Design review of the part built by this model. Coordinates are the model's own, in mm. Face numbers are marked on the shaded views. A direction names the side the tool comes from. Give positions to 0.01 mm unless a question says otherwise; leave off trailing zeros. Write each loop counter-clockwise with the first axis right and the second up, starting at its lowest first coordinate (ties: lowest second). Pieces come first, ordered by that corner, then holes. Notation, with made-up numbers: M 2.5,54 L 14.5,54 A14 ccw 14.5,63 Z; hole C 71,5.25 d3. An arc over 180 degrees is marked long. Use one line per item in the form item = value. Start each with the question number.
from build123d import *

# Parameters (mm, degrees)
SKETCH2_R           = 13.4112
BOSS_EXTRUDE1_DEPTH = 38.1
SKETCH5_W           = 26.8224
SKETCH5_H           = 184.15
BOSS_EXTRUDE2_DEPTH = 16.7386
SKETCH8_W           = 76.2
SKETCH8_H           = 38.1
BOSS_EXTRUDE3_DEPTH = 13.97
SKETCH9_W           = 1.016
SKETCH9_H           = 38.1
BOSS_EXTRUDE4_DEPTH = 38.1
SKETCH10_W          = 25.4
SKETCH10_H          = 38.1
BOSS_EXTRUDE5_DEPTH = 12.446
FILLET1_R           = 3.81


with BuildPart() as part:
    # Sketch2 → Boss-Extrude1 (new body)
    with BuildSketch(Plane.XY):
        with Locations(Location((0, 0, 0), (0, 0, 180))):
            Circle(SKETCH2_R)
    extrude(amount=BOSS_EXTRUDE1_DEPTH)

    # Sketch5 → Boss-Extrude2 (add)
    with BuildSketch(Plane.XY.offset(38.1)):
        with Locations((0, 92.075)):
            Rectangle(SKETCH5_W, SKETCH5_H)
    extrude(amount=-BOSS_EXTRUDE2_DEPTH)

    # Sketch8 → Boss-Extrude3 (add)
    with BuildSketch(Plane(origin=(0, 184.15, 0), x_dir=(1, 0, 0), z_dir=(0, 1, 0))):
        with Locations((0, -18.948214994)):
            Rectangle(SKETCH8_W, SKETCH8_H)
    extrude(amount=BOSS_EXTRUDE3_DEPTH)

    # Sketch9 → Boss-Extrude4 (add)
    with BuildSketch(Plane(origin=(0, 198.12, 0), x_dir=(1, 0, 0), z_dir=(0, 1, 0))):
        with Locations((-37.592, -18.948214994)):
            Rectangle(SKETCH9_W, SKETCH9_H)
        with Locations((37.592, -18.948214994)):
            Rectangle(SKETCH9_W, SKETCH9_H)
    extrude(amount=BOSS_EXTRUDE4_DEPTH)

    # Sketch10 → Boss-Extrude5 (add)
    with BuildSketch(Plane(origin=(0, 236.22, 0), x_dir=(1, 0, 0), z_dir=(0, 1, 0))):
        with Locations((-25.4, -18.948214994)):
            Rectangle(SKETCH10_W, SKETCH10_H)
        with Locations((25.4, -18.948214994)):
            Rectangle(SKETCH10_W, SKETCH10_H)
    extrude(amount=BOSS_EXTRUDE5_DEPTH)

    # Fillet1
    # the kernel refuses this fillet: 3.81 mm, written as the material it takes off along each edge
    with BuildSketch(Plane(origin=(15.598152153, 184.15, 38.1), x_dir=(0, 0, -1), z_dir=(-1, 0, 0))) as fillet1_piece_1:
        with BuildLine():
            CenterArc((3.81, 0.874780861), FILLET1_R, 180, 13.273598337)
            Line((0, 0.874780861), (-0.0762, 0.874780861))
            Line((-0.0762, 0.874780861), (-0.0762, 0))
            Line((-0.0762, 0), (0, -0.0762))
            ThreePointArc((0, -0.0762), (0.050892503, -0.0762), (0.027620706, -0.017495617))
            Line((0.027620706, -0.017495617), (0.101785006, 0))
        make_face()
    extrude(amount=31.196304306, mode=Mode.SUBTRACT)


solid = part.part
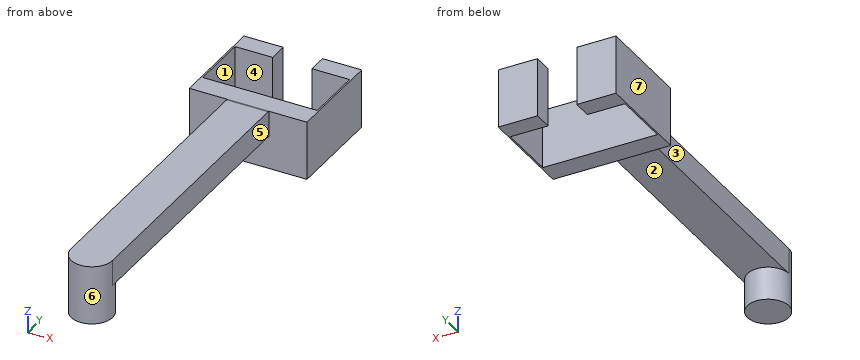
1. We need section B-B (z = 18). State the section outline as (x, y) points, and give its area (3 significant figures).
2. To check wall thickness, follow L1, parallel to Y at x = -23.5, z = 9.5; L2, parallel to X at y = 25, z = 31; L3, parallel to Y at x = 9, z = 11. State the ranges of each line that lie inside material, in increasing order.
3. For the marked faces 4, 5, 6 and 7, list the 3-axis set-ups (+Z, -Z, +X, -X, +Y, -Y) from which the entire face can be reached by the end or side of a thin tool; tool diameter is ignored.
4. We need section C-C (z = 32). State the section outline as (x, y) points.
5. We need section D-D (x = 0). State the section outline as (y, z) points.
6. We need section A-A (x = -28.5). State the section outline as (y, z) points, and give its area (3 significant figures).
7. Draft analysis for pull direction X (two halves, no side actions). For the marked faces 1, 2 and 3, state which applies: pulls with the +X half, pulls with the -X half, needs draft (parallel to the pull), parting line crosses it, or undercut.
8. Clearance check with flat-ended pins moving along their axes: pin 1 Ø6 at (y, z) = (60, 31.5) entering from +X; pin 2 Ø6 at (y, z) = (72, 24) entering from -X; pin 3 Ø12 at (x, z) = (31, 23.5) entering from -Y. State where each tip first meets the part, or that it passes through.
Answer block:
q1.outline = M -38.1,184.15 L 38.1,184.15 L 38.1,248.67 L 12.7,248.67 L 12.7,236.22 L 37.08,236.22 L 37.08,198.12 L -37.08,198.12 L -37.08,236.22 L -12.7,236.22 L -12.7,248.67 L -38.1,248.67 Z; C 0,0 d26.82
q1.area = 2,340 mm^2
q2.L1 = 184.15 to 198.12, 236.22 to 248.67
q2.L2 = -13.41 to 13.41
q2.L3 = -9.94 to 9.94, 184.15 to 198.12
q3.face_4 = +Z, -Z
q3.face_5 = +Z, -Z, +X, -Y
q3.face_6 = -Z
q3.face_7 = +Z, -Z, -X, +Y, -Y
q4.outline = M -38.1,184.15 L -13.41,184.15 L -13.41,0 A13.41 ccw 13.41,0 L 13.41,184.15 L 38.1,184.15 L 38.1,248.67 L 12.7,248.67 L 12.7,236.22 L 37.08,236.22 L 37.08,198.12 L -37.08,198.12 L -37.08,236.22 L -12.7,236.22 L -12.7,248.67 L -38.1,248.67 Z
q5.outline = M -13.41,0 L 13.41,0 L 13.41,21.36 L 184.15,21.36 L 184.15,-0.1 L 198.12,-0.1 L 198.12,38 L 184.15,38 A3.81 ccw 183.28,38.1 L -13.41,38.1 Z
q6.outline = M 184.15,-0.1 L 198.12,-0.1 L 198.12,38 L 184.15,38 Z; M 236.22,-0.1 L 248.67,-0.1 L 248.67,38 L 236.22,38 Z
q6.area = 1,010 mm^2
q7.face_1 = undercut
q7.face_2 = needs draft
q7.face_3 = pulls with the -X half
q8.pin_1 = 13.41
q8.pin_2 = -13.41
q8.pin_3 = 184.15
